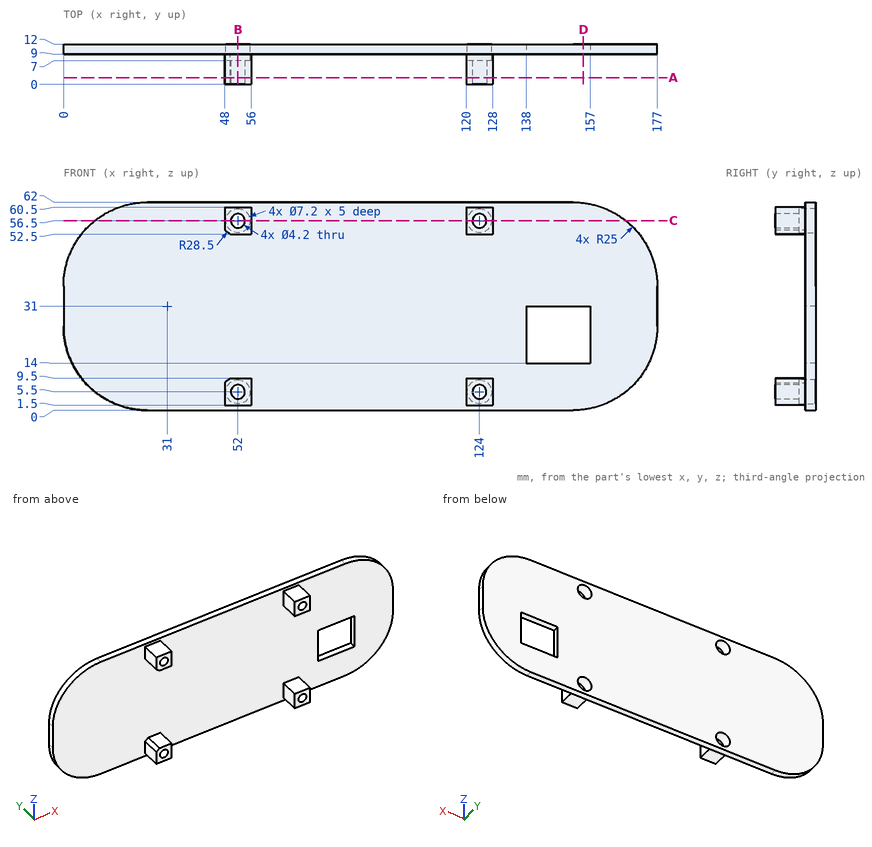
Study the drawing (mm; zero at the part's minimum x, y, z) and answer. Coordinates: 2 decimals unless noted, no trailing zeros. Loops run counter-clockwise (first coordinate to the right, second up) from the corner with the lowest first, then second, coordinate; pieces in that order, holes last. Notation, with made-up numbers: (-1, -6) -> (39, -6) arc R14 cw to (39, 2) -> close; hole circle Ø6 at (27.5, 60). An arc over 180 degrees is marked (long way). Write item = value, one per line. Start each with the question number.
1) The part is cut by section C-C, the plane z = 56.5. Determine the outline of the cut face in (x, y), plus the area to 3 significant figures.
2) Find the intervals of material crossed by L1, parallel to X at y = 6.5, z = 59; L2, parallel to X at y = 8.4, z = 56.5; L3, parallel to X at y = 1.75, z = 5.5, in increasing order. Write a range as from..to.
3) The part is cut by section D-D, the plane x = 155. Determine the outline of the cut face in (y, z), plus the area to 3 significant figures.
4) Given P1, Ø6.5, axis at x = 124, z = 5.5, coming from the -Y side; P2, Ø4, axis at x = 125.5, y = 3.5, coming from the +Z side; P3, Ø3.5, axis at y = 4.5, z = 58, coming from the -X side; P4, Ø6.5, axis at x = 123, y = 4.5, coming from the -Z side, each flat-ended and moving along its own axis, determine where each tip first touches the part or whether it passes through.
5) The part is cut by section B-B, the plane x = 52. Determine the outline of the cut face in (y, z), plus the area to 3 significant figures.
6) The part is cut by section A-A, the plane y = 2. Determine the outline of the cut face in (x, z).
Result:
q1.outline = (9.36, 9) -> (48, 9) -> (48, 0) -> (49.9, 0) -> (49.9, 7) -> (48.4, 7) -> (48.4, 12) -> (9.36, 12) -> close; (54.1, 0) -> (56, 0) -> (56, 9) -> (120, 9) -> (120, 0) -> (121.9, 0) -> (121.9, 7) -> (120.4, 7) -> (120.4, 12) -> (55.6, 12) -> (55.6, 7) -> (54.1, 7) -> close; (126.1, 0) -> (128, 0) -> (128, 9) -> (167.64, 9) -> (167.64, 12) -> (127.6, 12) -> (127.6, 7) -> (126.1, 7) -> close
q1.area = 488 mm²
q2.L1 = 48..56, 120..128
q2.L2 = 48..48.4, 55.6..56, 120..120.4, 127.6..128
q2.L3 = 48..49.9, 54.1..56, 120..121.9, 126.1..128
q3.outline = (9, 0.18) -> (12, 0.18) -> (12, 14) -> (9, 14) -> close; (9, 31) -> (12, 31) -> (12, 61.82) -> (9, 61.82) -> close
q3.area = 134 mm²
q4.P1 = 0
q4.P2 = 60.5
q4.P3 = 48
q4.P4 = 1.5
q5.outline = (0, 1.5) -> (9, 1.5) -> (9, 0) -> (12, 0) -> (12, 1.9) -> (7, 1.9) -> (7, 3.4) -> (0, 3.4) -> close; (0, 7.6) -> (7, 7.6) -> (7, 9.1) -> (12, 9.1) -> (12, 52.9) -> (7, 52.9) -> (7, 54.4) -> (0, 54.4) -> (0, 52.5) -> (9, 52.5) -> (9, 9.5) -> (0, 9.5) -> close; (0, 58.6) -> (7, 58.6) -> (7, 60.1) -> (12, 60.1) -> (12, 62) -> (9, 62) -> (9, 60.5) -> (0, 60.5) -> close
q5.area = 199 mm²
q6.outline = (48, 1.5) -> (56, 1.5) -> (56, 9.5) -> (49.71, 9.5) arc R28.5 cw to (48, 8.13) -> close; (48, 53.87) arc R28.5 cw to (49.71, 52.5) -> (56, 52.5) -> (56, 60.5) -> (48, 60.5) -> close; (120, 1.5) -> (128, 1.5) -> (128, 9.5) -> (120, 9.5) -> close; (120, 52.5) -> (128, 52.5) -> (128, 60.5) -> (120, 60.5) -> close; hole circle Ø4.2 at (52, 5.5); hole circle Ø4.2 at (52, 56.5); hole circle Ø4.2 at (124, 5.5); hole circle Ø4.2 at (124, 56.5)
